Part print with two shaded views. Sizes in mm from the minimum x, y, z corner. A direction names the side the tool comes from. Round coordinates to 2 decimals unless told otherwise and drop trailing zeros. Write each loop counter-clockwise with the first axis right and the second up, starting at its lowest first coordinate (ties: lowest second). Pieces come first, ordered by that corner, then holes. Notation, with made-up numbers: (5, -11) -> (49, -11) arc R30 ccw to (49, 20) -> close; hole circle Ø10 at (10.25, 1.5). An arc over 180 degrees is marked (long way). Answer in a Markdown table with one row per item.
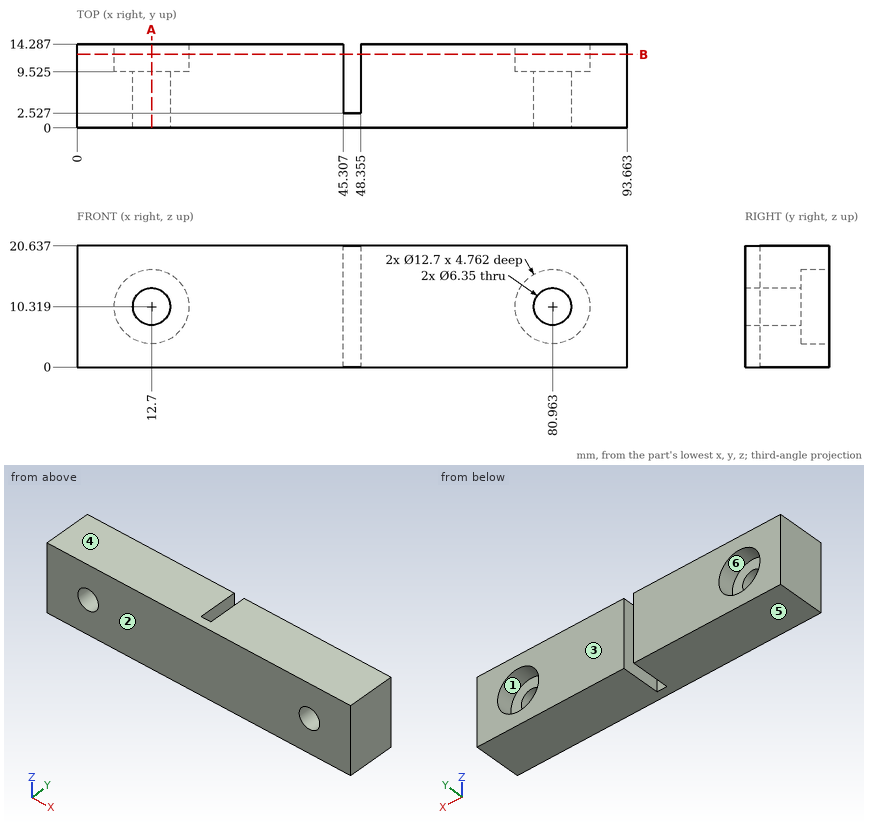
Q1. Two-plate mould, pull along Z, no slides. Class the marked faces 3, 4, 5 and 6: released by +Z, released by -Z, zero draft, split by the parting line, or undercut.
A:
| item | result |
|---|---|
| face 3 | zero draft |
| face 4 | released by +Z |
| face 5 | released by -Z |
| face 6 | undercut |
Q2. Saw through at B-B on y = 12.5. State how many separate pieces and enclosed holes the cut face has, plus the area to 3 significant figures.
A:
| item | result |
|---|---|
| separate pieces | 2 |
| enclosed holes | 2 |
| area | 1,620 mm² |
Q3. Saw through at A-A on x = 12.7. Write the cut outline in (y, z) (1 decimal).
A:
| item | result |
|---|---|
| outline | (0, 0) -> (14.3, 0) -> (14.3, 4) -> (9.5, 4) -> (9.5, 7.1) -> (0, 7.1) -> close; (0, 13.5) -> (9.5, 13.5) -> (9.5, 16.7) -> (14.3, 16.7) -> (14.3, 20.6) -> (0, 20.6) -> close |
Q4. Which spindle directions (+Z, -Z, +X, -X, +Y, -Y) get a long thin tool onto all of the face, cutting with end or side? Do the marked faces 1 and 2. Say none if no direction does.
A:
| item | result |
|---|---|
| face 1 | +Y |
| face 2 | +Z, -Z, +X, -X, -Y |
Q5. Wall check: line 1 (X direction, y = 5, z = 19) (1 decimal); line 2 (X direction, y = 11.5, z = 6) (1 decimal); line 3 (Z direction, x = 12.7, y = 5). Give the ranges that are in metal, low to high. Write a range as [from, to].
A:
| item | result |
|---|---|
| line 1 | [0, 45.3], [48.4, 93.7] |
| line 2 | [0, 8], [17.4, 45.3], [48.4, 76.3], [85.6, 93.7] |
| line 3 | [0, 7.14], [13.49, 20.64] |
Q6. Drop flat-ended pins along their axis: P1, Ø0.9, axis at x = 46.5, z = 10.5, coming from the +Y side; P2, Ø4, axis at x = 79, z = 9.5, coming from the +Y side (1 decimal). Give the stop position or say it passes through.
A:
| item | result |
|---|---|
| P1 | y = 2.53 |
| P2 | y = 9.5 |
